The model under review builds one solid part; all positions refer to its coordinate system, in mm. A direction names the side the tool comes from. Round coordinates to 2 decimals unless told otherwise and drop trailing zeros. Order: outer loops, then holes, each group sorted by start corner. A loop starts at its lowest first (then second) coordinate and runs counter-clockwise, first axis right, second up. Notation, with made-up numbers: M 66,65.5 L 71,65.5 A14 cw 71,71.5 Z; hole C 45.5,3 d7. An arc over 180 degrees is marked long. Answer as a JSON object with one key per item and string values. Group by question number.
1) The part is to be moulded in two halves that separate along Y. For faces 1 (the flat face through (0, 0, -2.5)), 2 (the flat face through (0, 0, 47)), 3 (the cylindrical face through (0.54, -2.44, -1.23)), say which applies: +Y half, -Y half, draft (parallel to the pull), parting line (faces both ways), or undercut.
2) Insertion check: pin 1 Ø2 at (x, z) = (1, 25.5) entering from -Y; pin 2 Ø2 at (x, z) = (-3.5, 35.5) entering from -Y; pin 3 Ø4 at (x, y) = (0, 0) entering from +Z; pin 4 Ø1.5 at (x, z) = (-2.5, 11.5) entering from +Y. Each pin has a flat end and moves straight along its axis. Give the tip position at first contact, or say it passes through.
3) Consider section D-D, the plane x = -4.5. Write out the cut boundary in (y, z).
4) For faces 4 (the flat face through (-2.5, 1.3, 50)), 5 (the cylindrical face through (2.45, -1.01, 48.52)), 6 (the flat face through (2.35, 1.29, 0)), list the 3-axis set-ups (+Z, -Z, +X, -X, +Y, -Y) from which the entire face can be reached by the end or side of a thin tool; tool diameter is ignored.
5) Consider section C-C, the plane z = 30. Write out the cut boundary in (x, y), then the cut area to 3 significant figures.
6) Consider section A-A, the plane y = 0. Write out the cut boundary in (x, z).
7) To check wall thickness, follow line 1 (Y direction, x = 0, z = 48.25); line 2 (Z direction, x = -2.5, y = -2.5); line 3 (X direction, y = 0.25, z = 7). State the ranges of each line that lie inside material, in increasing order.
```python
from build123d import *

# Parameters (mm, degrees)
SKETCH1_R           = 5.45
BOSS_EXTRUDE1_DEPTH = 50
SKETCH6_R           = 2.5
BOSS_EXTRUDE2_DEPTH = 2.5
SKETCH7_R           = 2.65
CUT_EXTRUDE1_DEPTH  = 3


with BuildPart() as part:
    # Sketch1 → Boss-Extrude1 (new body)
    with BuildSketch(Plane.XY):
        Circle(SKETCH1_R)
    extrude(amount=BOSS_EXTRUDE1_DEPTH)

    # Sketch6 → Boss-Extrude2 (add)
    with BuildSketch(Plane(origin=(0, 0, 0), x_dir=(-1, 0, 0), z_dir=(0, 0, -1))):
        Circle(SKETCH6_R)
    extrude(amount=BOSS_EXTRUDE2_DEPTH)

    # Sketch7 → Cut-Extrude1 (cut)
    with BuildSketch(Plane.XY.offset(50)):
        Circle(SKETCH7_R)
    extrude(amount=-CUT_EXTRUDE1_DEPTH, mode=Mode.SUBTRACT)


solid = part.part
```
Results list:
{
 "1": {"face 1": "draft", "face 2": "undercut", "face 3": "parting line"},
 "2": {"pin 1": "y = -5.45", "pin 2": "y = -4.84", "pin 3": "z = 47", "pin 4": "y = 5.16"},
 "3": {"outline": "M -3.07,0 L 3.07,0 L 3.07,50 L -3.07,50 Z"},
 "4": {"face 4": "+Z, +X, -X, +Y, -Y", "face 5": "+Z", "face 6": "-Z"},
 "5": {"outline": "C 0,0 d10.9", "area": "93.3 mm^2"},
 "6": {"outline": "M -5.45,0 L -2.5,0 L -2.5,-2.5 L 2.5,-2.5 L 2.5,0 L 5.45,0 L 5.45,50 L 2.65,50 L 2.65,47 L -2.65,47 L -2.65,50 L -5.45,50 Z"},
 "7": {"line 1": "-5.45 to -2.65, 2.65 to 5.45", "line 2": "0 to 50", "line 3": "-5.44 to 5.44"}
}
